from build123d import *

# Parameters (mm, degrees)
SKETCH_1_R      = 30
EXTRUDE_1_DEPTH = 2
EXTRUDE_2_DEPTH = 2
SKETCH_3_R      = 21.549788195
EXTRUDE_3_DEPTH = 1
CHAMFER_1_SIZE  = 1
CHAMFER_2_SIZE  = 1
CHAMFER_3_SIZE  = 1


with BuildPart() as part:
    # Эскиз1 → Бобышка-Вытянуть1 (new body)
    with BuildSketch(Plane.XY):
        with Locations((-49.331170663, 19.945627645)):
            Circle(SKETCH_1_R)
    extrude(amount=EXTRUDE_1_DEPTH)

    # Эскиз2 → Бобышка-Вытянуть2 (add)
    with BuildSketch(Plane.XY.offset(2)):
        Polygon((-20.825153864, 24.499783942), (-39.02217731, 46.909640502), (-67.528194109, 42.355484205), (-77.837187462, 15.391471347), (-59.640164016, -7.018385213), (-31.134147217, -2.464228916), align=None)
    extrude(amount=EXTRUDE_2_DEPTH)

    # Эскиз3 → Бобышка-Вытянуть3 (add)
    with BuildSketch(Plane.XY.offset(4)):
        with Locations((-49.331170663, 19.945627645)):
            Circle(SKETCH_3_R)
    extrude(amount=EXTRUDE_3_DEPTH)

    # Фаска1
    chamfer_1_edges = [part.edges().sort_by_distance(p)[0] for p in [
        (-25.97965054, 11.017777513, 4),
        (-29.923665587, 35.704712222, 4),
        (-53.275185709, 44.632562353, 4),
        (-72.682690785, 28.873477776, 4),
        (-68.738675739, 4.186543067, 4),
        (-45.387155617, -4.741307064, 4),
    ]]
    chamfer(chamfer_1_edges, length=CHAMFER_1_SIZE)

    # Фаска2
    chamfer_2_edges = [part.edges().sort_by_distance(p)[0] for p in [
        (-70.880958858, 19.945627645, 5),
    ]]
    chamfer(chamfer_2_edges, length=CHAMFER_2_SIZE - 0.0001)  # a hair under: the kernel refuses the full size

    # Фаска3
    chamfer_3_edges = [part.edges().sort_by_distance(p)[0] for p in [
        (-79.331170663, 19.945627645, 2),
    ]]
    chamfer(chamfer_3_edges, length=CHAMFER_3_SIZE)


solid = part.part
Model file for the job. Use its own axes, mm. A direction names the side the tool comes from. Give positions to 0.01 mm unless a question says otherwise; leave off trailing zeros.
1) Tool access for faces 1 (the flat face through (-45.587, -4.773, 2.493)), 2 (the flat face through (-72.61, 29.06, 2.49)), 3 (the flat face through (-68.866, 4.343, 2.493)), 4 (the flat face through (-68, 32, 4)): list every direction of +Z, -Z, +X, -X, +Y, -Y with a clear straight run to the whole face (end or side of a thin tool).
2) Flat gauge pins, fed straight in: pin 1 Ø1.5 at (y, z) = (26.5, 1.5) entering from -X; pin 2 Ø3 at (y, z) = (10, 1) entering from +X; pin 3 Ø1.5 at (y, z) = (35.5, 1.5) entering from -X; pin 4 Ø12 at (x, y) = (-26.5, 1) entering from -Z. Where does each tip first touch, or does it go through?
3) Wall check: line 1 (Z direction, x = -68, y = -1.5); line 2 (X direction, y = 12, z = 1.4); line 3 (Z direction, x = -28, y = 14). Give the ranges that are in metal, low to high.
Answer block:
1. face 1: +Z, +X, -Y
1. face 2: +Z, -X, +Y
1. face 3: +Z, -X, -Y
1. face 4: +Z
2. pin 1: stops at x = -78.73
2. pin 2: stops at x = -20.54
2. pin 3: stops at x = -75.31
2. pin 4: stops at z = 0
3. line 1: z = 0 to 2
3. line 2: x = -77.84 to -20.82
3. line 3: z = 0 to 4
